```python
from build123d import *

# Parameters (mm, degrees)
SKETCH1_R              = 9
BOSS_EXTRUDE1_DEPTH    = 4
SKETCH3_W              = 3
SKETCH3_H              = 2
CUT_EXTRUDE1_DEPTH     = 14.341664064
CIRPATTERN1_COUNT      = 4
M10X1_0_TAPPED_HOLE1_D = 9
SKETCH4_R              = 4.625
CUT_EXTRUDE2_DEPTH     = 14.171939872


with BuildPart() as part:
    # Sketch1 → Boss-Extrude1 (new body)
    with BuildSketch(Plane.XY):
        Circle(SKETCH1_R)
    extrude(amount=BOSS_EXTRUDE1_DEPTH)

    # Sketch3 → Cut-Extrude1 (cut, through all)
    with BuildSketch(Plane.XY.offset(4)):
        with Locations((0, 8)):
            Rectangle(SKETCH3_W, SKETCH3_H)
    cut_extrude1 = extrude(amount=-CUT_EXTRUDE1_DEPTH, mode=Mode.SUBTRACT)

    # CirPattern1: Cut-Extrude1 ×4 about axis
    cirpattern1_axis = Axis((0, 0, 0), (0, 0, 1))
    for i in range(1, CIRPATTERN1_COUNT):
        add(cut_extrude1.rotate(cirpattern1_axis, i * 360 / CIRPATTERN1_COUNT), mode=Mode.SUBTRACT)

    # Sketch2 → Cut-Revolve1 (revolve, cut)
    with BuildSketch(Plane(origin=(0, 0, 0), x_dir=(0, 0, -1), z_dir=(1, 0, 0)), mode=Mode.PRIVATE) as cut_revolve1_sk:
        Polygon((-1.227731474, 9), (0, 6.75), (0, 9), align=None)
    revolve(cut_revolve1_sk.sketch.rotate(Axis((0, 0, 4.2), (0, 0, -1)), 90), axis=Axis((0, 0, 4.2), (0, 0, -1)), mode=Mode.SUBTRACT)

    # M10x1.0 Tapped Hole1 (through all)
    with Locations(Plane.XY.offset(4)):
        with Locations((0, 0)):
            Hole(M10X1_0_TAPPED_HOLE1_D / 2)

    # Sketch4 → Cut-Extrude2 (cut, through all)
    with BuildSketch(Plane.XY.offset(4)):
        Circle(SKETCH4_R)
    extrude(amount=-CUT_EXTRUDE2_DEPTH, mode=Mode.SUBTRACT)


solid = part.part
```
The model under review builds one solid part; all positions refer to its coordinate system, in mm. A direction names the side the tool comes from. Give positions to 0.01 mm unless a question says otherwise; leave off trailing zeros. Write each loop counter-clockwise with the first axis right and the second up, starting at its lowest first coordinate (ties: lowest second). Pieces come first, ordered by that corner, then holes. Notation, with made-up numbers: M 0,10.5 L 17,10.5 A29 ccw 17,36.5 Z; hole C 33,7 d4. An arc over 180 degrees is marked long. Write each question's results on one line, items separated by ' | '. Start each with the question number.
1. We need section A-A (x = 0). Write out the cut boundary in (y, z) (3 decimals).
2. For probe 1 along Y at (x, z) = (0, 2.85) (3 decimals); probe 2 along X at (y, z) = (-4, 3); probe 3 along Y at (x, z) = (3, 1.8), list the stretches that pass through material, from the lowest coordinate up. Write a range as [from, to].
3. We need section D-D (z = 0.8). Write out the cut boundary in (x, y) (3 decimals).
4. Insertion check: pin 1 Ø2 at (x, z) = (-6.5, 1.5) entering from +Y; pin 2 Ø0.6 at (x, z) = (-8, 1.5) entering from +Y; pin 3 Ø1.5 at (x, z) = (-0.5, 3) entering from +Y. Each pin has a flat end and moves straight along its axis. Give the tip position at first contact, or say it passes through.
5. Mouldability with a two-part tool opening along X and no side actions: class faces 6 (the cylindrical face through (-6.42, -6.31, 2.59)), 7 (the flat face through (-8, 1.5, 3)), 8 (the flat face through (0, 7, 2)), 9 (the flat face through (-1.5, 8, 3)) as released by +X, released by -X, zero draft, split by the parting line, or undercut.
6. For faces 1 (the flat face through (1.5, -8, 3)), 2 (the flat face through (-8, -1.5, 3)), 3 (the flat face through (8, -1.5, 3)), 4 (the flat face through (1.5, 8, 3)), 5 (the cylindrical face through (6.42, 6.31, 2.59)), list the 3-axis set-ups (+Z, -Z, +X, -X, +Y, -Y) from which the entire face can be reached by the end or side of a thin tool; tool diameter is ignored.
7. We need section C-C (z = 2.6). Write out the cut boundary in (x, y) (3 decimals).
Results found:
1) outline: M -7,0.136 L -6.75,0 L -4.625,0 L -4.625,4 L -7,4 Z; M 4.625,0 L 6.75,0 L 7,0.136 L 7,4 L 4.625,4 Z
2) probe 1: y = [-7, -4.625], [4.625, 7] | probe 2: x = [-8.06, -2.32], [2.32, 8.06] | probe 3: y = [-8.49, -3.52], [3.52, 8.49]
3) outline: M -8.078,-1.5 A8.216 ccw -1.5,-8.078 L -1.5,-7 L 1.5,-7 L 1.5,-8.078 A8.216 ccw 8.078,-1.5 L 7,-1.5 L 7,1.5 L 8.078,1.5 A8.216 ccw 1.5,8.078 L 1.5,7 L -1.5,7 L -1.5,8.078 A8.216 ccw -8.078,1.5 L -7,1.5 L -7,-1.5 Z; hole C 0,0 d9.25
4) pin 1: stops at y = 7.12 | pin 2: stops at y = 4.66 | pin 3: stops at y = 7
5) face 6: released by -X | face 7: zero draft | face 8: undercut | face 9: undercut
6) face 1: +Z, -Z, -Y | face 2: +Z, -Z, -X | face 3: +Z, -Z, +X | face 4: +Z, -Z, +Y | face 5: +Z, -Z, +X, +Y
7) outline: M -8.874,-1.5 A9 ccw -1.5,-8.874 L -1.5,-7 L 1.5,-7 L 1.5,-8.874 A9 ccw 8.874,-1.5 L 7,-1.5 L 7,1.5 L 8.874,1.5 A9 ccw 1.5,8.874 L 1.5,7 L -1.5,7 L -1.5,8.874 A9 ccw -8.874,1.5 L -7,1.5 L -7,-1.5 Z; hole C 0,0 d9.25
